Part model, mm, in its own coordinate system. Face numbers are marked on the shaded views. Give positions to 0.01 mm unless a question says otherwise; leave off trailing zeros. Write each loop counter-clockwise with the first axis right and the second up, starting at its lowest first coordinate (ties: lowest second). Pieces come first, ordered by that corner, then holes. Notation, with made-up numbers: M 26,11.25 L 44,11.25 A11 cw 44,19.25 Z; hole C -30.5,38.25 d11. An arc over 180 degrees is marked long. Answer as CSV lines item,"result". Start each with the question number.
1) Wall check: line 1 along Y through (x, z) = (0, 9.5); line 2 along X through (y, z) = (0.5, 13.75) (3 decimals); line 3 along X through (y, z) = (13.5, 17.25). Give the ranges that are in metal, low to high. Write a range as from..to.
2) Mould opens along X. For the marked faces 1, 2 and 3 say: pulls with the +X half, pulls with the -X half, needs draft (parallel to the pull), parting line crosses it, or undercut.
3) Slice it at C-C, the plane z = 4.75. Give the cut face in (x, y), plus the area to 3 significant figures.
4) Slice it at D-D, the plane z = -0.75. Give the cut face in (x, y), plus the area to 3 significant figures.
5) Pin check, flat tips, straight feed: pin 1 Ø12 at (x, y) = (13.5, -21.5) entering from +Z; pin 2 Ø6 at (y, z) = (0, 7) entering from -X; pin 3 Ø1.5 at (y, z) = (-17, 15) entering from -X; pin 4 Ø10 at (x, z) = (-3, 11) entering from -Y. Stop position of each tip, or through.
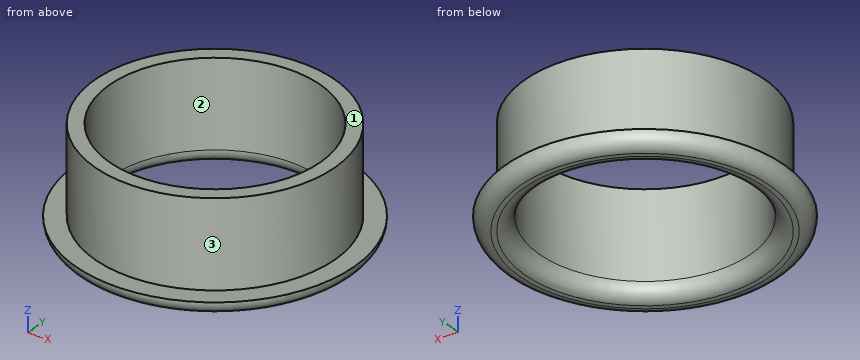
```python
from build123d import *

# Parameters (mm, degrees)
F0_R     = 25
F1_DEPTH = 18
F2_R     = 29
F3_DEPTH = 3
F4_R     = 22
F5_DEPTH = 21.001
F6_R     = 2.99999


# Not quite as in the source:
# - a fillet or chamfer is up to 0.001 mm smaller than in the source, because OpenCascade refuses the exact size


with BuildPart() as f1:
    # F0 (on Top) → F1 (new body)
    with BuildSketch(Plane.XY):
        Circle(F0_R)
    extrude(amount=F1_DEPTH)

    # F2 (on Top) → F3 (join)
    with BuildSketch(Plane.XY):
        Circle(F2_R)
    extrude(amount=-F3_DEPTH)

    # F4 (on face) → F5 (cut, through all)
    with BuildSketch(Plane.XY.offset(18)):
        Circle(F4_R)
    extrude(amount=-F5_DEPTH, mode=Mode.SUBTRACT)

    # F6 (radius 3 in the source; OpenCascade refuses exactly that, so slightly less here)
    f6_edges = [f1.edges().sort_by_distance(p)[0] for p in [
        (-22, 0, -3),
        (-29, 0, -3),
    ]]
    fillet(f6_edges, radius=F6_R)


solid = f1.part
```
Found:
1,line 1,"-25..-22, 22..25"
1,line 2,"-24.995..-21.994, 21.994..24.995"
1,line 3,"-21.04..-17.37, 17.37..21.04"
2,face 1,"needs draft"
2,face 2,"undercut"
2,face 3,"parting line crosses it"
3,outline,"C 0,0 d50; hole C 0,0 d44"
3,area,"443 mm²"
4,outline,"C 0,0 d57.81; hole C 0,0 d44.19"
4,area,"1,090 mm²"
5,pin 1,"z = 18"
5,pin 2,"x = -25"
5,pin 3,"x = -19"
5,pin 4,"y = -25"
